Part print with two shaded views. Sizes in mm from the minimum x, y, z corner. Give positions to 0.01 mm unless a question says otherwise; leave off trailing zeros. Write each loop counter-clockwise with the first axis right and the second up, starting at its lowest first coordinate (ties: lowest second). Pieces come first, ordered by that corner, then holes.
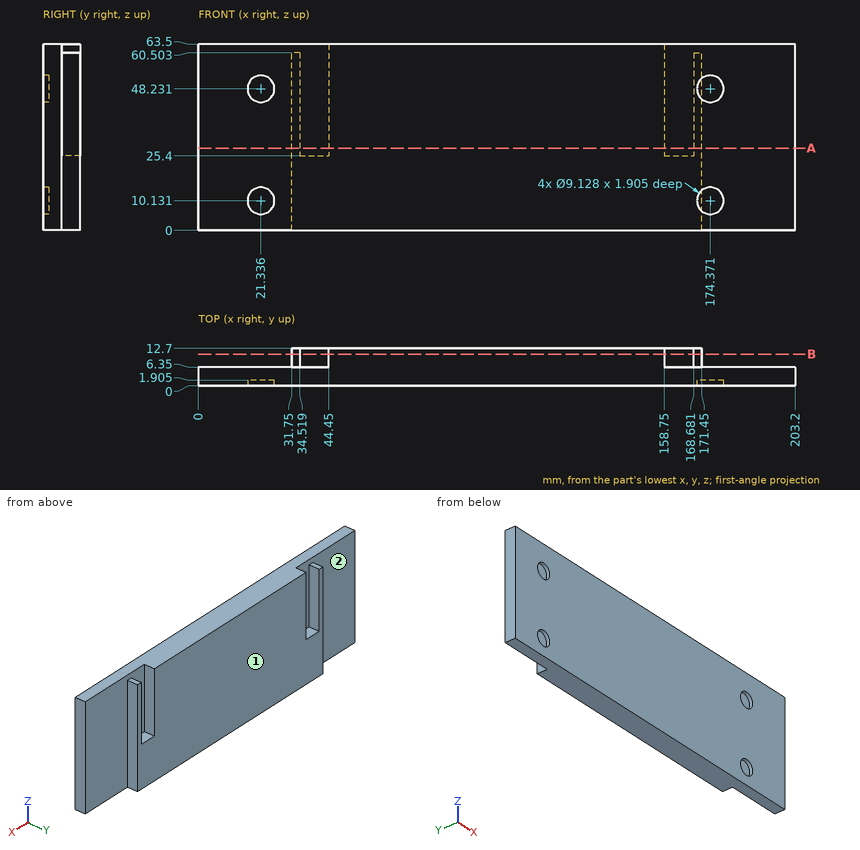
1) Saw through at B-B, the plane y = 10.75. Write the cut outline in (x, z), then the cut area to 3 significant figures.
Answers follow:
outline: (31.75, 0) - (171.45, 0) - (171.45, 60.5) - (168.68, 60.5) - (168.68, 25.4) - (158.75, 25.4) - (158.75, 63.5) - (44.45, 63.5) - (44.45, 25.4) - (34.52, 25.4) - (34.52, 60.5) - (31.75, 60.5) - close
area: 8,100 mm2
2) Pin check, flat tips, straight feed: pin 1 Ø2 at (x, y) = (169.5, 10) entering from +Z; pin 2 Ø13.5 at (x, z) = (24, 43) entering from +Y; pin 3 Ø7.5 at (x, z) = (174.5, 9.5) entering from -Y (3 decimals). Stop position of each tip, or through.
Answers follow:
pin 1: stops at z = 60.5
pin 2: stops at y = 6.35
pin 3: stops at y = 1.905
3) Wall check: L1, parallel to X at y = 8.5, z = 46.5; L2, parallel to X at y = 8.25, z = 17.5; L3, parallel to Z at x = 43, y = 7. Give the ranges that are in metal, low to high.
Answers follow:
L1: x = 31.75 to 34.52, 44.45 to 158.75, 168.68 to 171.45
L2: x = 31.75 to 171.45
L3: z = 0 to 25.4
4) Saw through at A-A, the plane z = 28. Write the cut outline in (x, y).
Answers follow:
outline: (0, 0) - (203.2, 0) - (203.2, 6.35) - (171.45, 6.35) - (171.45, 12.7) - (168.68, 12.7) - (168.68, 6.35) - (158.75, 6.35) - (158.75, 12.7) - (44.45, 12.7) - (44.45, 6.35) - (34.52, 6.35) - (34.52, 12.7) - (31.75, 12.7) - (31.75, 6.35) - (0, 6.35) - close
5) Two-plate mould, pull along X, no slides. Class the marked faces 1 and 2: +X half, -X half, draft (parallel to the pull), parting line (faces both ways), or undercut.
Answers follow:
face 1: draft
face 2: undercut
